from build123d import *

# Parameters (mm, degrees)
F0_W     = 75
F0_H     = 75
F1_DEPTH = 900
F2_W     = 50
F2_H     = 50
F3_DEPTH = 50
F5_W     = 50
F5_H     = 50
F6_DEPTH = 50


with BuildPart() as f1:
    # F0 (on Top) → F1 (new body)
    with BuildSketch(Plane.XY):
        Rectangle(F0_W, F0_H)
    extrude(amount=F1_DEPTH)

    # F2 (on face) → F3 (cut)
    with BuildSketch(Plane.YZ.offset(37.5)):
        with Locations((1.5, 162.5)):
            Rectangle(F2_W, F2_H)
    extrude(amount=-F3_DEPTH, mode=Mode.SUBTRACT)

    # F5 (on face) → F6 (cut)
    with BuildSketch(Plane(origin=(0, 37.5, 0), x_dir=(-1, 0, 0), z_dir=(0, 1, 0))):
        with Locations((-1.5, 162.5)):
            Rectangle(F5_W, F5_H)
    extrude(amount=-F6_DEPTH, mode=Mode.SUBTRACT)


solid = f1.part
Can you work these out from the model? Positions are in its coordinate system, mm. A direction names the side the tool comes from. Give positions to 0.01 mm unless a question says otherwise; leave off trailing zeros. Loops run counter-clockwise (first coordinate to the right, second up) from the corner with the lowest first, then second, coordinate; pieces in that order, holes last. Notation, with made-up numbers: (25.25, 60) - (72.25, 60) arc R22 cw to (72.25, 80) - close; hole circle Ø10 at (2.5, 1). An arc over 180 degrees is marked (long way). Return JSON: item names as keys, results as strings.
1. We'd pull the mould along Z, two halves only. Please class faces 4 (the face through (-1, -37.5, 444)), 5 (the face through (-1, 1, 900)), 6 (the face through (13, -23.5, 162)): +Z half, -Z half, draft (parallel to the pull), parting line (faces both ways), or undercut.
Output values:
{"face 4": "draft", "face 5": "+Z half", "face 6": "undercut"}
2. I'm going to push flat-ended pins straight in: pin 1 Ø12 at (x, z) = (-17, 156) entering from +Y; pin 2 Ø12 at (y, z) = (-15.5, 156) entering from +X. Where does each tip first touch, or does it pass through?
Output values:
{"pin 1": "stops at y = -12.5", "pin 2": "stops at x = -12.5"}
3. For faces 1 (the face through (7, 7, 187.5)), 2 (the face through (-1, 1, 0)), 3 (the face through (-23.5, 13, 162)), which set-ups out of +Z, -Z, +X, -X, +Y, -Y let a thin tool reach every point of the face, with its end or its side?
Output values:
{"face 1": "none", "face 2": "-Z, +X, -X, +Y, -Y", "face 3": "+Y"}
4. I want a section at A-A on x = 11.5. Please give me the cut outline in (y, z).
Output values:
{"outline": "(-37.5, 0) - (37.5, 0) - (37.5, 137.5) - (-23.5, 137.5) - (-23.5, 187.5) - (37.5, 187.5) - (37.5, 900) - (-37.5, 900) - close"}
5. If I drill on line 1 (Z direction, x = -11.5, y = -15); line 2 (Y direction, x = -20, z = 162.5); line 3 (Y direction, x = 12.5, z = 163.5), over which ranges is the centre line in solid material (lowest first)?
Output values:
{"line 1": "z = 0 to 137.5, 187.5 to 900", "line 2": "y = -37.5 to -12.5", "line 3": "y = -37.5 to -23.5"}
